Answer from the drawing. Dimensions are ordinates in mm from the lowest x, y and z of the part. A direction names the side the tool comes from. Coordinates: 2 decimals unless noted, no trailing zeros. Write each loop counter-clockwise with the first axis right and the second up, starting at its lowest first coordinate (ties: lowest second). Pieces come first, ordered by that corner, then holes.
1) Find the intervals of material crossed by line 1 (Y direction, x = 29, z = 84.5); line 2 (X direction, y = 25, z = 62.5), in increasing order.
2) The part is cut by section A-A (y = 78). Determine the outline of the cut face in (x, z) (1 decimal).
3) The part is cut by section B-B (z = 19). Determine the outline of the cut face in (x, y) (1 decimal), then the cut area to 3 significant figures.
4) Which of the six approach directions +Z, -Z, +X, -X, +Y, -Y give full straight-line access (tool end or side, diameter ignored) to the marked faces 1, 2 and 3?
5) Each of these flat-tipped pins is pushed along its axis until it touches: pin 1 Ø12 at (x, z) = (55, 32) entering from +Y; pin 2 Ø3 at (y, z) = (30.5, 48.5) entering from -X. Where does it stop, or does it pass through?
6) The part is cut by section C-C (z = 34.5). Determine the outline of the cut face in (x, y).
7) The part is cut by section D-D (x = 17). Determine the outline of the cut face in (y, z).
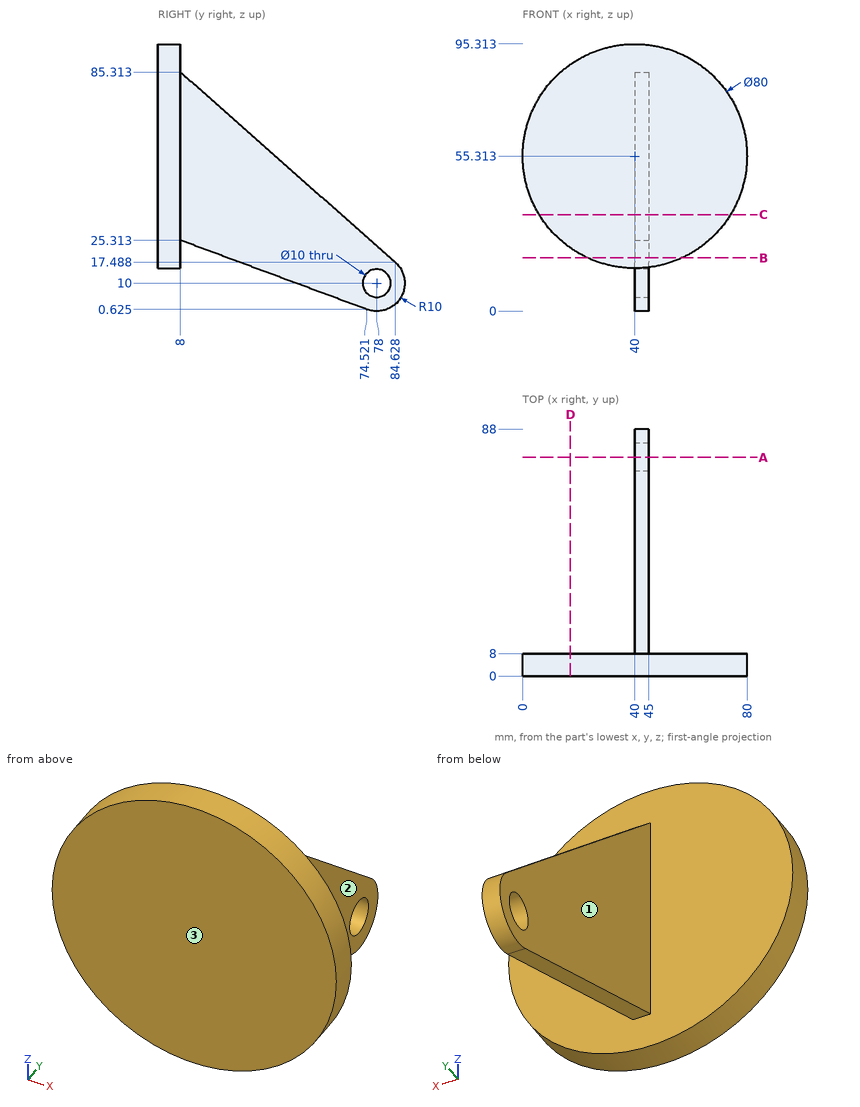
Reported:
1. line 1: y = 0 to 8
1. line 2: x = 40 to 45
2. outline: (40, 0) - (45, 0) - (45, 5) - (40, 5) - close; (40, 15) - (45, 15) - (45, 23.4) - (40, 23.4) - close
3. outline: (23.2, 0) - (56.8, 0) - (56.8, 8) - (23.2, 8) - close; (40, 25) - (45, 25) - (45, 82.9) - (40, 82.9) - close
3. area: 558 mm2
4. face 1: +Z, -Z, -X, +Y
4. face 2: +Z, -Z, +X, +Y
4. face 3: +Z, -Z, +X, -X, -Y
5. pin 1: stops at y = 8
5. pin 2: stops at x = 40
6. outline: (5.84, 0) - (74.16, 0) - (74.16, 8) - (45, 8) - (45, 65.41) - (40, 65.41) - (40, 8) - (5.84, 8) - close
7. outline: (0, 22.59) - (8, 22.59) - (8, 88.04) - (0, 88.04) - close
